The listing builds one solid part. Answer for the finished solid, in the listing's coordinates (mm). A direction names the side the tool comes from. Give positions to 0.01 mm unless a question says otherwise; leave off trailing zeros. Order: outer loops, then holes, each group sorted by start corner. A loop starts at its lowest first (then second) coordinate and runs counter-clockwise, first axis right, second up.
Autodesk Inventor part; units mm, degrees
ref_plane "MSC_PF1" through (0, 0, 0) normal (1, 0, 0) x (0, 1, 0)
ref_plane "MSC_PT1" through (0, 0, 0) normal (0, 0, -1) x (-1, 0, 0)
ref_plane "YZ Plane" through (0, 0, 0) normal (1, 0, 0) x (0, 1, 0)
sketch "Эскиз2" plane through (0, 0, 0) normal (0, 0, 1) x (1, 0, 0)
  circle A0 centre (0, 0) radius 2.5
  dimension "d3" = 5
extrude "Выдавливание1" add sketch "Эскиз2" against normal blind 1.87
sketch "Эскиз3" plane through (0, 0, -1.87) normal (0, 0, -1) x (-1, 0, 0)
  circle A0 centre (0, 0) radius 3
  circle A1 centre (0, 0) radius 2.5 construction
  dimension "d28" = 360
  dimension "d9" = 6
extrude "Выдавливание2" add sketch "Эскиз3" along normal blind 28.13
chamfer "Фаска1" distance 0.5 distance2 0.5 1 edges at (3, 0, -1.87) measured on face at (-2.7801, -0.4387, -1.87)
sketch "Эскиз4" plane through (0, 0, 0) normal (0, 0, 1) x (1, 0, 0)
  circle A0 centre (0, 0) radius 6.2
  circle A1 centre (0, 0) radius 2.5 construction
  dimension "d15" = 12.4
extrude "Выдавливание3" add sketch "Эскиз4" along normal blind 2.4
fillet "Сопряжение1" radius 0.25 1 edges at (-2.5, 0, 0)
sketch "Эскиз5" plane through (0, 0, 0) normal (0, 1, 0) x (-1, 0, 0)
  line L0 (6.2, 2.4) -> (6.2, 0)
  line L1 (5.99, 2.4) -> (6.2, 2.4)
  line L2 (6.2, 0) -> (5.99, 2.4)
  line L3 (-6.2, 2.4) -> (6.2, 2.4) construction
  line L4 (-6.2, 0) -> (6.2, 0) construction
  line L5 (0, -0.48) -> (0, 2.88)
  line L6 (8.68, 0) -> (-8.68, 0)
  dimension "d20" = 5
  dimension "d56" = 6.2
  dimension "d57" = 2.4
revolve "Вращение1" cut sketch "Эскиз5" angle 360 about axis through (0, 0, -10) along (0, 0, 1)
sketch "Эскиз6" plane through (0, 0, 0) normal (0, 1, 0) x (-1, 0, 0)
  line L0 (0, 3.7) -> (0, 2.4)
  arc A0 (5.99, 2.4) -> (0, 3.7) centre (-2.2245, -21) ccw
  line L1 (0, 2.4) -> (5.99, 2.4)
  line L2 (5.99, 2.4) -> (-5.99, 2.4) construction
  line L3 (0, -4.4495) -> (0, 0.4495)
  line L4 (0, -25.9772) -> (0, 8.8629)
  line L5 (8.4344, 0) -> (-8.3941, 0)
  dimension "d58" = 1.3
  dimension "d59" = 5.99
  dimension "d60" = 0
  dimension "d62" = 24.8
revolve "Вращение2" add sketch "Эскиз6" angle 360 about axis through (0, 0, -4.4495) along (0, 0, 1)
sketch "Эскиз7" plane through (0, 0, 0) normal (0, 1, 0) x (-1, 0, 0)
  line L0 (3.15, 3.7) -> (-3.15, 3.7)
  line L1 (1.8164, 0.84) -> (3.15, 3.7)
  line L2 (-1.8164, 0.84) -> (1.8164, 0.84)
  line L3 (-3.15, 3.7) -> (-1.8164, 0.84)
  line L4 (0, 0.268) -> (0, 4.272)
  line L5 (4.41, 0) -> (-4.41, 0)
  dimension "d32" = 2.86
  dimension "d34" = 65
  dimension "d36" = 65
  dimension "d63" = 3.15
  dimension "d64" = 3.7
  dimension "d65" = 6.3
extrude "Выдавливание4" cut sketch "Эскиз7" against normal mid plane 2.1
sketch "Эскиз8" plane through (0, 0, 0) normal (1, 0, 0) x (0, 1, 0)
  line L0 (-1.8164, 0.84) -> (-3.15, 3.7)
  line L1 (1.8164, 0.84) -> (-1.8164, 0.84)
  line L2 (3.15, 3.7) -> (1.8164, 0.84)
  line L3 (-3.15, 3.7) -> (3.15, 3.7)
  line L4 (0, 0.268) -> (0, 4.272)
  line L5 (-4.41, 0) -> (4.41, 0)
  dimension "d40" = 65
  dimension "d42" = 65
  dimension "d44" = 2.86
  dimension "d66" = 6.3
  dimension "d67" = 3.7
  dimension "d69" = 3.15
extrude "Выдавливание5" cut sketch "Эскиз8" along normal mid plane 2.1
sketch "Эскиз9" plane through (0, 0, 0) normal (0, 1, 0) x (-1, 0, 0)
  line L0 (0, 3.7) -> (0, 0.84)
  line L1 (2.52, 3.7) -> (0, 3.7)
  line L2 (0, 0.84) -> (2.52, 3.7)
  line L3 (-6.2, 0) -> (6.2, 0) construction
  line L4 (0, -0.74) -> (0, 4.44)
  line L5 (8.68, 0) -> (-8.68, 0)
  dimension "d50" = 2.86
  dimension "d52" = 2.86
  dimension "d54" = 2.52
  dimension "d70" = 0
  dimension "d71" = 3.7
revolve "Вращение3" cut sketch "Эскиз9" angle 360 about axis through (0, 0, -10) along (0, 0, 1)
thread "Резьба1"
ref_plane "MSC_PF1" through (0, 0, 0) normal (1, 0, 0) x (0, 1, 0)
ref_plane "MSC_PT1" through (0, 0, 0) normal (0, 0, -1) x (-1, 0, 0)
equation "\"d4\" = -b + NLG"
equation "\"d9\" = NND"
equation "\"d10\" = b"
equation "\"d12\" = -0.5 * msp_ds + 0.5 * NND"
equation "\"d13\" = 0.5 * NND - 0.5 * msp_ds"
equation "\"d15\" = Dk"
equation "\"d16\" = ParK"
equation "\"d18\" = r"
equation "\"d32\" = q"
equation "\"d63\" = 0.5 * M"
equation "\"d64\" = ParK + ParF"
equation "\"d65\" = M"
equation "\"d37\" = 2 * msp_s"
equation "\"d44\" = q"
equation "\"d66\" = M"
equation "\"d67\" = ParK + ParF"
equation "\"d69\" = 0.5 * M"
equation "\"d47\" = 2 * msp_s"
equation "\"d3\" = msp_ds"
equation "\"d56\" = 0.5 * Dk"
equation "\"d57\" = ParK"
equation "\"d58\" = ParF"
equation "\"d59\" = 0.5 * Dk - msp_v"
equation "\"d62\" = 2 * Dk"
equation "\"d50\" = q"
equation "\"d52\" = q"
equation "\"d54\" = msp_rr"
equation "\"d71\" = ParK + ParF"
equation "\"PTC\" = 1"
equation "\"NLG\" = 30"
equation "\"Dk\" = 12.4"
equation "\"ParK\" = 2.4"
equation "\"NND\" = 6"
equation "\"M\" = 6.3"
equation "\"q\" = 2.86"
equation "\"r\" = 0.25"
equation "\"msp_ds\" = NND - PTC"
equation "\"b\" = 28.13"
equation "\"msp_x\" = 1.25 * PTC"
equation "\"msp_s\" = 0.166667 * M"
equation "\"msp_rr\" = 0.4 * M"
equation "\"ParF\" = 1.3"
equation "\"msp_v\" = 0.0874887 * ParK"
equation "\"THREADDIA\" = NND"
properties part number "JIS B 1111 - M6x30" material "Сталь, мягкая"
1) Find section A-A (z = -16.5). Write down the section's boundary in (x, y), then the cut area to 3 significant figures.
Geometry says:
outline: circle Ø6 at (0, 0)
area: 28.3 mm2
2) Straight lines are drawn through the part: probe 1 along Z at (x, y) = (0.5, -4); probe 2 along Z at (x, y) = (2.75, 0.75); probe 3 along X at (y, z) = (-0.5, 1.5). For each, find the intervals that lie inside material, in ascending order.
Geometry says:
probe 1: z = 0 to 3
probe 2: z = -30 to -2.22, 0 to 2.84
probe 3: x = -6.05 to -2.12, 2.12 to 6.05
3) A tool of negligible diameter and unlimited length cuts with its end or side. For faces 1 (the cylindrical face through (-0.54, -2.44, -1.05)), 2 (the flat face through (-2, 1.05, 2)), from which of +Z, -Z, +X, -X, +Y, -Y can it reach the whole face along a straight path? Write none if from no direction.
Geometry says:
face 1: none
face 2: +Z
4) For a pull along X with two mould halves and no side action, classify faces 3 (the cylindrical face through (3, 0, -16)), 4 (the flat face through (1.05, 2, 2)), 5 (the flat face through (0, 0, -30)) as +X half, -X half, draft (parallel to the pull), parting line (faces both ways), or undercut.
Geometry says:
face 3: parting line
face 4: undercut
face 5: draft
5) Given P1, Ø1, axis at x = 3, y = -4.5, coming from the +Z side; P2, Ø2, axis at y = -2.5, z = 1.5, coming from the -X side; P3, Ø0.6, axis at y = -2, z = 2, coming from the +X side, each flat-ended and moving along its own axis, determine where each tip first touches the part or whether it passes through.
Geometry says:
P1: stops at z = 2.75
P2: stops at x = -5.9
P3: stops at x = 5.78
